from build123d import *

# Parameters (mm, degrees)
SKETCH_1_W          = 50
SKETCH_1_H          = 8
EXTRUDE_1_DEPTH     = 1.5
SKETCH_2_R          = 2.1
CUT_EXTRUDE_1_DEPTH = 26.362373706
CHAMFER_1_SIZE      = 1


with BuildPart() as part:
    # 草图1 → 凸台-拉伸1 (new body)
    with BuildSketch(Plane(origin=(0, 0, 0), x_dir=(1, 0, 0), z_dir=(0, 1, 0))):
        Rectangle(SKETCH_1_W, SKETCH_1_H)
    extrude(amount=EXTRUDE_1_DEPTH)

    # 草图2 → 切除-拉伸1 (cut, through all)
    with BuildSketch(Plane(origin=(0, 1.5, 0), x_dir=(1, 0, 0), z_dir=(0, 1, 0))):
        with Locations(Location((-20, 0, 0), (0, 0, 270))):
            Circle(SKETCH_2_R)
        with Locations(Location((20, 0, 0), (0, 0, 90))):
            Circle(SKETCH_2_R)
    extrude(amount=-CUT_EXTRUDE_1_DEPTH, mode=Mode.SUBTRACT)

    # 倒角1
    chamfer_1_edges = [part.edges().sort_by_distance(p)[0] for p in [
        (25, 0.75, 4),
        (-25, 0.75, 4),
        (-25, 0.75, -4),
        (25, 0.75, -4),
    ]]
    chamfer(chamfer_1_edges, length=CHAMFER_1_SIZE)


solid = part.part
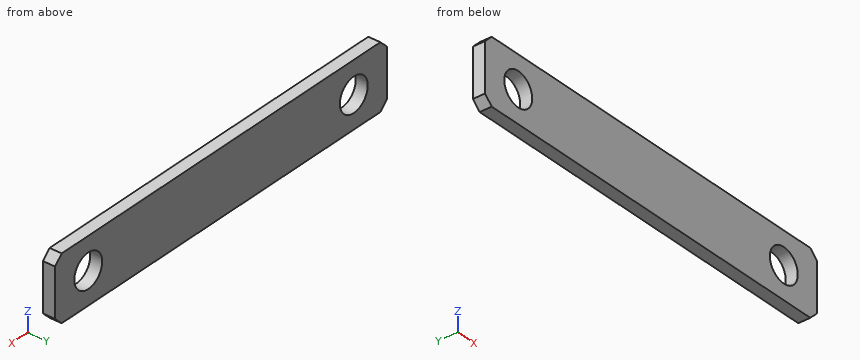
Part model, mm, in its own coordinate system. Round coordinates to 2 decimals unless told otherwise and drop trailing zeros. Order: outer loops, then holes, each group sorted by start corner. A loop starts at its lowest first (then second) coordinate and runs counter-clockwise, first axis right, second up. Notation, with made-up numbers: (76.25, 19) -> (108.25, 19) arc R12 ccw to (108.25, 25) -> close; hole circle Ø9 at (73, 88.5). An arc over 180 degrees is marked (long way). Put each result on its own line as item: value.
Q1. Band-saw the part on B-B (z = 0). Give the cut face in (x, y).
From the geometry:
outline: (-25, 0) -> (-22.1, 0) -> (-22.1, 1.5) -> (-25, 1.5) -> close; (-17.9, 0) -> (17.9, 0) -> (17.9, 1.5) -> (-17.9, 1.5) -> close; (22.1, 0) -> (25, 0) -> (25, 1.5) -> (22.1, 1.5) -> close
Q2. Pin check, flat tip, straight feed: pin 1 Ø1 at (x, z) = (18, 2.5) entering from -Y. Stop position of the tip, or through.
From the geometry:
pin 1: stops at y = 0
Q3. Band-saw the part on C-C (x = -20). Give the cut face in (y, z), and give its area (3 significant figures).
From the geometry:
outline: (0, -4) -> (1.5, -4) -> (1.5, -2.1) -> (0, -2.1) -> close; (0, 2.1) -> (1.5, 2.1) -> (1.5, 4) -> (0, 4) -> close
area: 5.70 mm2
Q4. Band-saw the part on A-A (y = 1). Give the cut face in (x, z), and give its area (3 significant figures).
From the geometry:
outline: (-25, -3) -> (-24, -4) -> (24, -4) -> (25, -3) -> (25, 3) -> (24, 4) -> (-24, 4) -> (-25, 3) -> close; hole circle Ø4.2 at (-20, 0); hole circle Ø4.2 at (20, 0)
area: 370 mm2
Q5. Wall check: line 1 (X direction, y = 0.75, z = 0); line 2 (Z direction, x = 20, y = 0.5); line 3 (X direction, y = 0.55, z = 1.75). Give the ranges that are in metal, low to high. Write a range as [from, to].
From the geometry:
line 1: x = [-25, -22.1], [-17.9, 17.9], [22.1, 25]
line 2: z = [-4, -2.1], [2.1, 4]
line 3: x = [-25, -21.16], [-18.84, 18.84], [21.16, 25]
